Design review of the part built by this model. Coordinates are the model's own, in mm. Face numbers are marked on the shaded views. A direction names the side the tool comes from. Round coordinates to 2 decimals unless told otherwise and drop trailing zeros. Loops run counter-clockwise (first coordinate to the right, second up) from the corner with the lowest first, then second, coordinate; pieces in that order, holes last. Notation, with made-up numbers: M 9,-12.5 L 29,-12.5 A26 ccw 29,19.5 Z; hole C 28.5,20 d4. An arc over 180 degrees is marked long. Answer as CSV lines item,"result". Start each with the question number.
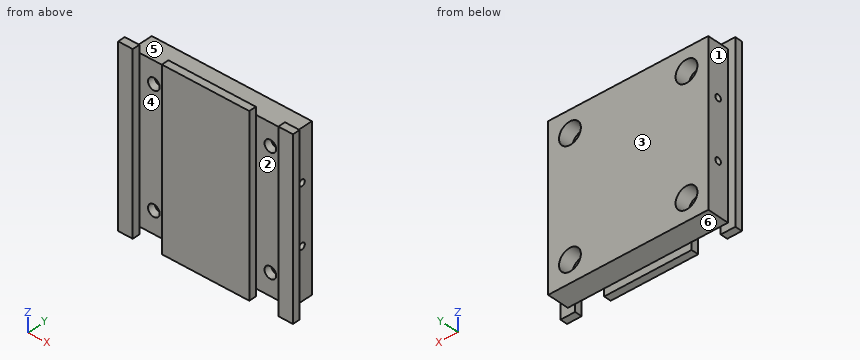
from build123d import *

# Parameters (mm, degrees)
SKETCH1_W           = 76.2
SKETCH1_H           = 76.2
BOSS_EXTRUDE1_DEPTH = 3.175
SKETCH2_W           = 69.79412
SKETCH2_H           = 69.79412
SKETCH2_W_2         = 57.09412
SKETCH2_H_2         = 57.09412
BOSS_EXTRUDE2_DEPTH = 9.525
SKETCH13_W          = 12.7
SKETCH13_H          = 76.2
CUT_EXTRUDE1_DEPTH  = 3.175
SKETCH15_R          = 2.5527
CUT_EXTRUDE2_DEPTH  = 55.716959208
SKETCH17_R          = 4.7625
CUT_EXTRUDE3_DEPTH  = 6.35


with BuildPart() as part:
    # Sketch1 → Boss-Extrude1 (new body)
    with BuildSketch(Plane(origin=(0, 0, 0), x_dir=(1, 0, 0), z_dir=(0, 1, 0))):
        Rectangle(SKETCH1_W, SKETCH1_H)
    extrude(amount=BOSS_EXTRUDE1_DEPTH)

    # Sketch2 → Boss-Extrude2 (add)
    # profile 1 of 2: a face of its own
    with BuildSketch(Plane(origin=(0, 3.175, 0), x_dir=(1, 0, 0), z_dir=(0, 1, 0))):
        Rectangle(SKETCH2_W, SKETCH2_H)
        Rectangle(SKETCH2_W_2, SKETCH2_H_2, mode=Mode.SUBTRACT)
    # profile 2 of 2: a face of its own
    with BuildSketch(Plane(origin=(0, 3.175, 0), x_dir=(1, 0, 0), z_dir=(0, 1, 0))):
        Rectangle(SKETCH2_W_2, SKETCH2_H_2)
    extrude(amount=BOSS_EXTRUDE2_DEPTH)

    # Sketch9 → #6-32 Tapped Hole2 (revolve, cut)
    with BuildSketch(Plane(origin=(34.89706, 7.9375, 12.7), x_dir=(0, 0, -1), z_dir=(0, 1, 0))):
        Polygon((0, 0), (0, 11.98869403), (1.35255, 11.176), (1.35255, 0), align=None)
    f_6_32_tapped_hole2 = revolve(axis=Axis((41.24706, 7.9375, 12.7), (-1, 0, 0)), mode=Mode.SUBTRACT)

    # Mirror1: #6-32 Tapped Hole2 across plane
    add(f_6_32_tapped_hole2.mirror(Plane.XY), mode=Mode.SUBTRACT)

    # Mirror2: #6-32 Tapped Hole2 across plane
    add(f_6_32_tapped_hole2.mirror(Plane(origin=(0, 0, 0), x_dir=(0, 0, 1), z_dir=(1, 0, 0))), mode=Mode.SUBTRACT)

    # Mirror2 copy 1 sketch → Mirror2 copy 1 (revolve, cut)
    with BuildSketch(Plane(origin=(-34.89706, 7.9375, -12.7), x_dir=(0, 0, 1), z_dir=(0, 1, 0))):
        Polygon((0, 0), (0, 11.98869403), (1.35255, 11.176), (1.35255, 0), align=None)
    revolve(axis=Axis((-41.24706, 7.9375, -12.7), (1, 0, 0)), mode=Mode.SUBTRACT)

    # Sketch13 → Cut-Extrude1 (cut)
    with BuildSketch(Plane.XZ):
        with Locations((-25.4, 0)):
            Rectangle(SKETCH13_W, SKETCH13_H)
        with Locations((25.4, 0)):
            Rectangle(SKETCH13_W, SKETCH13_H)
    extrude(amount=-CUT_EXTRUDE1_DEPTH, mode=Mode.SUBTRACT)

    # Sketch15 → Cut-Extrude2 (cut, through all)
    with BuildSketch(Plane.XZ.offset(-3.175)):
        with Locations(Location((-25.4, 25.4, 0), (0, 0, 270))):
            Circle(SKETCH15_R)
        with Locations(Location((25.4, 25.4, 0), (0, 0, 270))):
            Circle(SKETCH15_R)
        with Locations(Location((25.4, -25.4, 0), (0, 0, 270))):
            Circle(SKETCH15_R)
        with Locations(Location((-25.4, -25.4, 0), (0, 0, 270))):
            Circle(SKETCH15_R)
    extrude(amount=-CUT_EXTRUDE2_DEPTH, mode=Mode.SUBTRACT)

    # Sketch17 → Cut-Extrude3 (cut)
    with BuildSketch(Plane(origin=(0, 12.7, 0), x_dir=(1, 0, 0), z_dir=(0, 1, 0))):
        with Locations(Location((-25.4, 25.4, 0), (0, 0, 270))):
            Circle(SKETCH17_R)
        with Locations(Location((25.4, 25.4, 0), (0, 0, 270))):
            Circle(SKETCH17_R)
        with Locations(Location((25.4, -25.4, 0), (0, 0, 270))):
            Circle(SKETCH17_R)
        with Locations(Location((-25.4, -25.4, 0), (0, 0, 270))):
            Circle(SKETCH17_R)
    extrude(amount=-CUT_EXTRUDE3_DEPTH, mode=Mode.SUBTRACT)


solid = part.part
Item 1: Consider section C-C, the plane y = 11.75. Write out the cut boundary in (x, z) (1 decimal), then the cut area to 3 significant figures.
Item 2: To check wall thickness, follow line 1 (X direction, y = 11, z = 25); line 2 (X direction, y = 2, z = 29); line 3 (Y direction, x = 29.5, z = 12.7) (3 decimals). State the ranges of each line that lie inside material, in increasing order.
Item 3: Insertion check: pin 1 Ø8.5 at (x, z) = (-25.4, 25.4) entering from -Y (3 decimals); pin 2 Ø3.5 at (y, z) = (7.94, -12.7) entering from +X; pin 3 Ø5 at (x, y) = (-17.5, 11) entering from -Z. Each pin has a flat end and moves straight along its axis. Give the tip position at first contact, or say it passes through.
Item 4: Tool access review of the marked faces 4, 5 and 6: name each direction out of +Z, -Z, +X, -X, +Y, -Y from which nothing blocks a thin tool from reaching the whole face with its end or side.
Item 5: Consider section B-B, the plane z = 25.4. Count the separate pieces of the cut face and the enclosed holes in it, then the cut area to 3 significant figures.
Item 6: Consider section A-A, the plane y = 1. Write out the cut boundary in (x, z).
Item 7: The part is to be moulded in two halves that separate along X. For the marked faces 1, 2 and 3, say which applies: +X half, -X half, draft (parallel to the pull), parting line (faces both ways), or undercut.
Found:
1,outline,"M -34.9,-34.9 L 34.9,-34.9 L 34.9,34.9 L -34.9,34.9 Z; hole C -25.4,-25.4 d9.5; hole C -25.4,25.4 d9.5; hole C 25.4,-25.4 d9.5; hole C 25.4,25.4 d9.5"
1,area,"4,590 mm^2"
2,line 1,"x = -34.9 to -30.15, -20.65 to 20.65, 30.15 to 34.9"
2,line 2,"x = -38.1 to -31.75, -19.05 to 19.05, 31.75 to 38.1"
2,line 3,"y = 3.175 to 6.585, 9.29 to 12.7"
3,pin 1,"stops at y = 3.175"
3,pin 2,"stops at x = 34.9"
3,pin 3,"stops at z = -34.9"
4,face 4,"+Z, -Z, -Y"
4,face 5,"+Z, +X, -X, +Y"
4,face 6,"-Z, +X, -X, +Y"
5,separate pieces,"3"
5,enclosed holes,"0"
5,area,"673 mm^2"
6,outline,"M -38.1,-38.1 L -31.75,-38.1 L -31.75,38.1 L -38.1,38.1 Z; M -19.05,-38.1 L 19.05,-38.1 L 19.05,38.1 L -19.05,38.1 Z; M 31.75,-38.1 L 38.1,-38.1 L 38.1,38.1 L 31.75,38.1 Z"
7,face 1,"-X half"
7,face 2,"undercut"
7,face 3,"draft"
